Verification items for the finished model (mm, model axes). Face numbers are marked on the shaded views. A direction names the side the tool comes from. Coordinates: 2 decimals unless noted, no trailing zeros. Loops run counter-clockwise (first coordinate to the right, second up) from the corner with the lowest first, then second, coordinate; pieces in that order, holes last. Notation, with made-up numbers: (79.25, -32) - (133.25, -32) arc R14 cw to (133.25, -16) - close; hole circle Ø10 at (84, 60.5). An arc over 180 degrees is marked (long way). One line per item, written item: value. Start each with the question number.
(1) Draft check along Y on the marked faces 1, 2 and 3. Enter one of: +Y half, -Y half, draft (parallel to the pull), parting line (faces both ways), or undercut.
(2) Gauge pin test, flat ends, axial feed: P1, Ø0.7, axis at y = -42, z = 13.5, coming from the +X side; P2, Ø2.5, axis at y = -42, z = 13.5, coming from the -X side; P3, Ø4, axis at x = 18, y = 30, coming from the +Z side. Record the tip position at first contact, or that the pin passes through.
(3) Thickness scan on probe 1 along Y at (x, z) = (27, 10.5); probe 2 along X at (y, z) = (10, -7); probe 3 along Z at (x, y) = (-6, 19). Record the ranges inside material, lowest first. Write a range as [from, to].
(4) Section check A-A (z = 1). Record the boundary of the cut face in (x, y), plus the area to 3 significant figures.
(5) Section check C-C (y = -10.5). Record the boundary of the cut face in (x, z), plus the area to 3 significant figures.
(6) Section check D-D (x = -22). Record the boundary of the cut face in (y, z).
(7) Set-up check for the marked faces 4 and 5: record each of +Z, -Z, +X, -X, +Y, -Y from which the full face is reachable in a straight line by a thin tool's end or side.
(8) Section check B-B (x = 11). Record the boundary of the cut face in (y, z).
```python
from build123d import *

# Parameters (mm, degrees)
F1_DEPTH = 43.18
F2_W     = 57.685676
F2_H     = 78.818068
F3_DEPTH = 33.782
F4_W     = 20.835391
F4_H     = 2.243813
F5_DEPTH = 2.54


with BuildPart() as f1:
    # F0 (on Front) → F1 (new body, symmetric)
    with BuildSketch(Plane.XZ):
        with BuildLine():
            ThreePointArc((-39.37, -12.180453), (-37.510128, -16.670581), (-33.02, -18.530453))
            Line((-33.02, -18.530453), (33.02, -18.530453))
            ThreePointArc((33.02, -18.530453), (37.510128, -16.670581), (39.37, -12.180453))
            Line((39.37, -12.180453), (39.37, 9.409547))
            ThreePointArc((39.37, 9.409547), (37.510128, 13.899675), (33.02, 15.759547))
            Line((33.02, 15.759547), (-33.02, 15.759547))
            ThreePointArc((-33.02, 15.759547), (-37.510128, 13.899675), (-39.37, 9.409547))
            Line((-39.37, 9.409547), (-39.37, -12.180453))
        make_face()
    extrude(amount=F1_DEPTH, both=True)

    # F2 (on face) → F3 (cut)
    with BuildSketch(Plane.XY.offset(15.759547)):
        Rectangle(F2_W, F2_H)
    extrude(amount=-F3_DEPTH, mode=Mode.SUBTRACT)

    # F4 (on face) → F5 (cut)
    with BuildSketch(Plane.XZ.offset(43.18)):
        with Locations((-17.922866, 13.451327)):
            Rectangle(F4_W, F4_H)
    extrude(amount=-F5_DEPTH, mode=Mode.SUBTRACT)


solid = f1.part
```
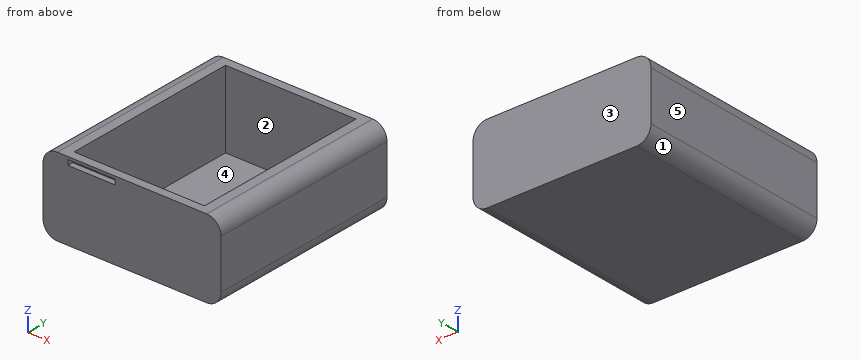
Responses:
1. face 1: draft
1. face 2: undercut
1. face 3: +Y half
2. P1: stops at x = 38.15
2. P2: stops at x = -38.7
2. P3: stops at z = -18.02
3. probe 1: y = [-43.18, -39.41], [39.41, 43.18]
3. probe 2: x = [-39.37, -28.84], [28.84, 39.37]
3. probe 3: z = [-18.53, -18.02]
4. outline: (-39.37, -43.18) - (39.37, -43.18) - (39.37, 43.18) - (-39.37, 43.18) - close; hole (-28.84, -39.41) - (28.84, -39.41) - (28.84, 39.41) - (-28.84, 39.41) - close
4. area: 2,250 mm²
5. outline: (-39.37, -12.18) arc R6.35 ccw to (-33.02, -18.53) - (33.02, -18.53) arc R6.35 ccw to (39.37, -12.18) - (39.37, 9.41) arc R6.35 ccw to (33.02, 15.76) - (28.84, 15.76) - (28.84, -18.02) - (-28.84, -18.02) - (-28.84, 15.76) - (-33.02, 15.76) arc R6.35 ccw to (-39.37, 9.41) - close
5. area: 717 mm²
6. outline: (-43.18, -18.53) - (43.18, -18.53) - (43.18, 15.76) - (39.41, 15.76) - (39.41, -18.02) - (-39.41, -18.02) - (-39.41, 15.76) - (-43.18, 15.76) - (-43.18, 14.57) - (-40.64, 14.57) - (-40.64, 12.33) - (-43.18, 12.33) - close
7. face 4: +Z
7. face 5: +Z, -Z, -X, +Y, -Y
8. outline: (-43.18, -18.53) - (43.18, -18.53) - (43.18, 15.76) - (39.41, 15.76) - (39.41, -18.02) - (-39.41, -18.02) - (-39.41, 15.76) - (-43.18, 15.76) - close
